```python
from build123d import *

# Parameters (mm, degrees)
RIBCUT1_DEPTH    = 0.508
RIBCUT2_DEPTH    = 0.8128
RIBCUTSPAT_COUNT = 12
RIBCUTSPAT_ANGLE = 330


with BuildPart() as part:
    # BodySke → BaseBody (revolve)
    with BuildSketch(Plane.XY, mode=Mode.PRIVATE) as basebody_sk:
        with BuildLine():
            Line((0, 0), (0, 4.36626))
            Line((0, 4.36626), (0.00508, 4.36626))
            Line((0.00508, 4.36626), (0.00508, 4.37134))
            ThreePointArc((0.00508, 4.37134), (0.40894, 4.7752), (0.8128, 4.37134))
            Line((0.8128, 4.37134), (0.8128, 4.3053))
            Line((0.8128, 4.3053), (1.6256, 4.1402))
            Line((1.6256, 4.1402), (1.6256, 3.9751))
            Line((1.6256, 3.9751), (18.20418, 3.9751))
            Line((18.20418, 3.9751), (19.05, 3.12928))
            Line((19.05, 3.12928), (19.05, 0))
            Line((19.05, 0), (0, 0))
        make_face()
    revolve(basebody_sk.sketch.rotate(Axis((0, 0, 0), (1, 0, 0)), 90), axis=Axis((0, 0, 0), (1, 0, 0)))

    # RibCut1Ske → RibCut1 (cut)
    with BuildSketch(Plane(origin=(1.6256, 0, 0), x_dir=(0, 0, -1), z_dir=(1, 0, 0))):
        with BuildLine():
            Line((0.518854667, 3.941092468), (0.518854667, 4.746927941))
            ThreePointArc((0.518854667, 4.746927941), (1.235912704, 4.612489006), (1.924122648, 4.37038752))
            Line((1.924122648, 4.37038752), (1.521204912, 3.67251353))
            ThreePointArc((1.521204912, 3.67251353), (1.028831586, 3.839651752), (0.518854667, 3.941092468))
        make_face()
    ribcut1 = extrude(amount=-RIBCUT1_DEPTH, mode=Mode.SUBTRACT)

    # RibCut2Ske → RibCut2 (cut)
    with BuildSketch(Plane(origin=(1.6256, 0, 0), x_dir=(0, 0, -1), z_dir=(1, 0, 0))):
        with BuildLine():
            Line((0.518854667, 4.107559601), (0.518854667, 4.746927941))
            ThreePointArc((0.518854667, 4.746927941), (1.235912704, 4.612489006), (1.924122648, 4.37038752))
            Line((1.924122648, 4.37038752), (1.604438478, 3.816678295))
            ThreePointArc((1.604438478, 3.816678295), (1.071562611, 3.999126106), (0.518854667, 4.107559601))
        make_face()
    ribcut2 = extrude(amount=-RIBCUT2_DEPTH, mode=Mode.SUBTRACT)

    # RibCutsPat: RibCut1, RibCut2 ×12 about axis
    ribcutspat_axis = Axis((0, 0, 0), (1, 0, 0))
    add([ribcut1.rotate(ribcutspat_axis, i * RIBCUTSPAT_ANGLE / (RIBCUTSPAT_COUNT - 1)) for i in range(1, RIBCUTSPAT_COUNT)], mode=Mode.SUBTRACT)
    add([ribcut2.rotate(ribcutspat_axis, i * RIBCUTSPAT_ANGLE / (RIBCUTSPAT_COUNT - 1)) for i in range(1, RIBCUTSPAT_COUNT)], mode=Mode.SUBTRACT)


solid = part.part
```
Read the model definition and answer for the solid it produces. Units are mm, in the model's axes. Coordinates: 2 decimals unless noted, no trailing zeros. Loops run counter-clockwise (first coordinate to the right, second up) from the corner with the lowest first, then second, coordinate; pieces in that order, holes last.
(1) Consider line 1 along Z through (x, y) = (3.5, -0.5); line 2 along Y through (x, z) = (9.75, -2). Determine where each line is inside the solid, lowest interval first.
Solution:
line 1: z = -3.94 to 3.94
line 2: y = -3.44 to 3.44
(2) Flat-ended cylindrical pins translate along their axes: pin 1 Ø0.5 at (y, z) = (-1.5, -4) entering from +X; pin 2 Ø3 at (x, z) = (9.5, 0) entering from -Y; pin 3 Ø0.5 at (y, z) = (-2, -3.5) entering from +X. Find the tip coordinate at first contact, or state that the pin passes through.
Solution:
pin 1: stops at x = 1.63
pin 2: stops at y = -3.98
pin 3: stops at x = 18.4
(3) The part is cut by section C-C (x = 2.75). Determine the outline of the cut face in (y, z).
Solution:
outline: circle Ø7.95 at (0, 0)
